Geometry check sheet. Reference: drawing and pictorial views, mm from the part's lowest x, y, z. A direction names the side the tool comes from. Coordinates: 2 decimals unless noted, no trailing zeros. Loops run counter-clockwise (first coordinate to the right, second up) from the corner with the lowest first, then second, coordinate; pieces in that order, holes last. Notation, with made-up numbers: (-16.75, -29) - (7.25, -29) arc R27 ccw to (7.25, -6) - close; hole circle Ø6 at (11.5, 80). An arc over 180 degrees is marked (long way). Write each question's results on one line, items separated by ' | '. Start each with the question number.
1. Cross-section at A-A (x = 17.5). Record the cut outline in (y, z).
2. Cross-section at D-D (x = 59). Record the cut outline in (y, z), and give its area (3 significant figures).
3. Thickness scan on line 1 (X direction, y = 18.5, z = 8); line 2 (Z direction, x = 14.5, y = 14.25); line 3 (Y direction, x = 4, z = 50.5). Record the ranges inside material, lowest first. Write a range as [from, to].
4. Cross-section at C-C (x = 39). Record the cut outline in (y, z), and give its area (3 significant figures).
5. Cross-section at B-B (z = 8). Record the cut outline in (x, y), and give its area (3 significant figures).
6. Tool access check on the marked faces 1 and 2. Record the directions out of +Z, -Z, +X, -X, +Y, -Y that give a thin tool (end or side, any length) a straight path to the whole face; none if there is none.
7. Gauge pin test, flat ends, axial feed: P1, Ø14.5, axis at x = 60, z = 8, coming from the -Y side; P2, Ø8.5, axis at x = 34.5, y = 7.5, coming from the -Z side; P3, Ø1.6, axis at x = 17, z = 62.5, coming from the +Y side. Record the tip position at first contact, or that the pin passes through.
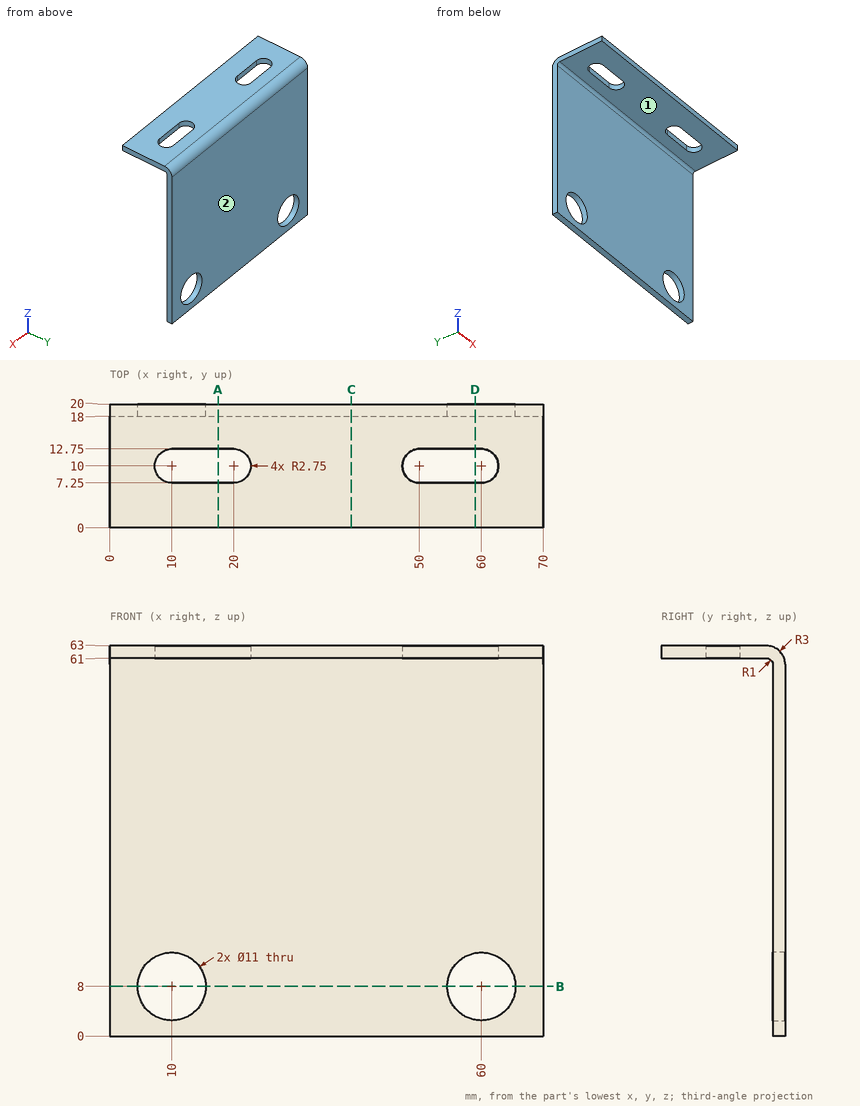
Established:
1) outline: (0, 61) - (7.25, 61) - (7.25, 63) - (0, 63) - close; (12.75, 61) - (17, 61) arc R1 cw to (18, 60) - (18, 0) - (20, 0) - (20, 60) arc R3 ccw to (17, 63) - (12.75, 63) - close
2) outline: (0, 61) - (7.25, 61) - (7.25, 63) - (0, 63) - close; (12.75, 61) - (17, 61) arc R1 cw to (18, 60) - (18, 13.41) - (20, 13.41) - (20, 60) arc R3 ccw to (17, 63) - (12.75, 63) - close; (18, 0) - (20, 0) - (20, 2.59) - (18, 2.59) - close | area: 128 mm^2
3) line 1: [0, 4.5], [15.5, 54.5], [65.5, 70] | line 2: [61, 63] | line 3: [18, 20]
4) outline: (0, 61) - (17, 61) arc R1 cw to (18, 60) - (18, 0) - (20, 0) - (20, 60) arc R3 ccw to (17, 63) - (0, 63) - close | area: 160 mm^2
5) outline: (0, 18) - (4.5, 18) - (4.5, 20) - (0, 20) - close; (15.5, 18) - (54.5, 18) - (54.5, 20) - (15.5, 20) - close; (65.5, 18) - (70, 18) - (70, 20) - (65.5, 20) - close | area: 96.0 mm^2
6) face 1: -Z, +X, -X, -Y | face 2: +Z, -Z, +X, -X, +Y
7) P1: y = 18 | P2: z = 61 | P3: y = 19.47
